Input: part model. Units: mm. Frame: model coordinates. Face numbers are marked on the shaded views. A direction names the side the tool comes from. Round coordinates to 2 decimals unless told otherwise and drop trailing zeros. Order: outer loops, then holes, each group sorted by start corner. A loop starts at its lowest first (then second) coordinate and runs counter-clockwise, first axis right, second up. Notation, with made-up numbers: (-19, 0.5) -> (14, 0.5) arc R14 ccw to (14, 26.5) -> close; hole circle Ø11 at (69.5, -1). An arc over 180 degrees is marked (long way). Use a Markdown table: item, result.
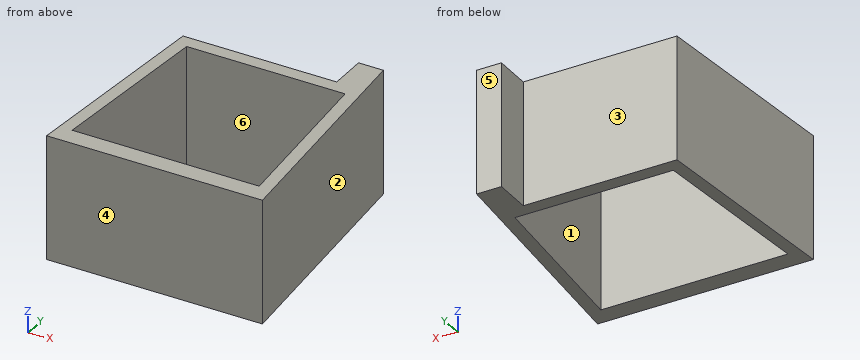
from build123d import *

# Parameters (mm, degrees)
F1_DEPTH = 20


# Not quite as in the source:
# - a feature names something its author has since deleted; it is built from what else it names


with BuildPart() as f1:
    # F0 (on Top) → F1 (new body)
    with BuildSketch(Plane.XY):
        Polygon((0, 15.9851339135), (-10.1, 15.9851339135), (-14.6001070377, 15.9851339135), (-17.3394622729, -16.880093272), (0, -16.880093272), (17.3394622729, -16.880093272), (14.1, 21.9851339135), (10.1, 21.9851339135), (10.1, 15.9851339135), align=None)
        Polygon((11.9072113089, -13.8146081649), (-11.9072113089, -13.8146081649), (-15.0287533179, -13.8146081649), (-12.7284283152, 13.7833838166), (-9.6068863062, 13.7833838166), (0, 13.7833838166), (9.6068863062, 13.7833838166), (12.7284283152, 13.7833838166), (15.0287533179, -13.8146081649), align=None, mode=Mode.SUBTRACT)
    extrude(amount=F1_DEPTH)


solid = f1.part
1) Cut plane B-B on x = 1. Return loops of the section in (y, z), and give its area (3 significant figures).
Answer key:
| item | result |
|---|---|
| outline | (-16.88, 0) -> (-13.81, 0) -> (-13.81, 20) -> (-16.88, 20) -> close; (13.78, 0) -> (15.99, 0) -> (15.99, 20) -> (13.78, 20) -> close |
| area | 105 mm^2 |
2) Cut plane C-C on y = 6. Return loops of the section in (x, z).
Answer key:
| item | result |
|---|---|
| outline | (-15.43, 0) -> (-13.38, 0) -> (-13.38, 20) -> (-15.43, 20) -> close; (13.38, 0) -> (15.43, 0) -> (15.43, 20) -> (13.38, 20) -> close |
3) Contact query for flat-ended pins moving along their axis: P1, Ø3, axis at y = -13, z = 14, coming from the -X side; P2, Ø5, axis at y = 20, z = 7.5, coming from the -X side; P3, Ø6, axis at x = -1, z = 6.5, coming from the +Y side. Output: stop coordinate, or through.
Answer key:
| item | result |
|---|---|
| P1 | stops at x = -17.14 |
| P2 | stops at x = 10.1 |
| P3 | stops at y = 15.99 |
4) Cut plane D-D on y = 18. Return loops of the section in (x, z), and give its area (3 significant figures).
Answer key:
| item | result |
|---|---|
| outline | (10.1, 0) -> (14.43, 0) -> (14.43, 20) -> (10.1, 20) -> close |
| area | 86.6 mm^2 |
5) Set-up query: the marked faces 1, 2 and 3. Return all of +Z, -Z, +X, -X, +Y, -Y with unobstructed straight access to the full face (end or side cutting, diameter ignored); none if empty.
Answer key:
| item | result |
|---|---|
| face 1 | +Z, -Z |
| face 2 | +Z, -Z, +X, +Y |
| face 3 | +Z, -Z, -X, +Y |
6) Draft query along Y for the marked faces 4, 5 and 6. Return one class per face: released by +Y, released by -Y, zero draft, split by the parting line, or undercut.
Answer key:
| item | result |
|---|---|
| face 4 | released by -Y |
| face 5 | released by +Y |
| face 6 | undercut |
7) Ray query, probe 1 along Y at (x, z) = (3.5, 6.75); probe 2 along X at (y, z) = (1.5, 12.5); probe 3 along X at (y, z) = (3, 2.25). Return the intervals inside material, ascending.
Answer key:
| item | result |
|---|---|
| probe 1 | y = -16.88 to -13.81, 13.78 to 15.99 |
| probe 2 | x = -15.81 to -13.75, 13.75 to 15.81 |
| probe 3 | x = -15.68 to -13.63, 13.63 to 15.68 |
8) Cut plane A-A on z = 16.5. Return loops of the section in (x, y), and give its area (3 significant figures).
Answer key:
| item | result |
|---|---|
| outline | (-17.34, -16.88) -> (17.34, -16.88) -> (14.1, 21.99) -> (10.1, 21.99) -> (10.1, 15.99) -> (-14.6, 15.99) -> close; hole (-15.03, -13.81) -> (15.03, -13.81) -> (12.73, 13.78) -> (-12.73, 13.78) -> close |
| area | 309 mm^2 |
